```python
from build123d import *

# Parameters (mm, degrees)
SKETCH_1_W          = 20
SKETCH_1_H          = 12
SKETCH_1_R          = 1.25
SKETCH_1_R_2        = 0.6
SKETCH_1_R_3        = 2.6
EXTRUDE_1_DEPTH     = 2.8
EXTRUDE_START       = 2.8
SKETCH_1_9_W        = 20
SKETCH_1_9_H        = 12
SKETCH_1_9_R        = 1.25
EXTRUDE_2_DEPTH     = 0.5
EXTRUDE_START_2     = 3.3
SKETCH_1_10_W       = 20
SKETCH_1_10_H       = 12
SKETCH_1_10_R       = 1.25
SKETCH_1_10_R_2     = 2.6
EXTRUDE_3_DEPTH     = 2.8
SKETCH_3_R          = 0.75
SKETCH_3_R_2        = 0.35
CUT_EXTRUDE_3_DEPTH = 25.108297327
CUT_EXTRUDE_START   = 6.1
SKETCH_3_4_R        = 1
CUT_EXTRUDE_5_DEPTH = 5.1


with BuildPart() as part:
    # 草图1 → 凸台-拉伸1 (new body)
    with BuildSketch(Plane(origin=(0, 0, 0), x_dir=(1, 0, 0), z_dir=(0, 1, 0))):
        with Locations((10, -6)):
            Rectangle(SKETCH_1_W, SKETCH_1_H)
        with Locations(Location((15, -6, 0), (0, 0, 270))):
            Circle(SKETCH_1_R, mode=Mode.SUBTRACT)
        with Locations(Location((7.678736094, -8.970584613, 0), (0, 0, 270))):
            Circle(SKETCH_1_R_2, mode=Mode.SUBTRACT)
        with Locations(Location((9.847079862, -3.807418404, 0), (0, 0, 270))):
            Circle(SKETCH_1_R_3, mode=Mode.SUBTRACT)
    extrude(amount=EXTRUDE_1_DEPTH)

    # 草图1<9> → 凸台-拉伸2 (add)
    with BuildSketch(Plane(origin=(0, 0, 0), x_dir=(1, 0, 0), z_dir=(0, 1, 0)).offset(EXTRUDE_START)):
        with Locations((10, -6)):
            Rectangle(SKETCH_1_9_W, SKETCH_1_9_H)
        with Locations(Location((15, -6, 0), (0, 0, 270))):
            Circle(SKETCH_1_9_R, mode=Mode.SUBTRACT)
    extrude(amount=EXTRUDE_2_DEPTH)

    # 草图1<10> → 凸台-拉伸3 (add)
    with BuildSketch(Plane(origin=(0, 0, 0), x_dir=(1, 0, 0), z_dir=(0, 1, 0)).offset(EXTRUDE_START_2)):
        with Locations((10, -6)):
            Rectangle(SKETCH_1_10_W, SKETCH_1_10_H)
        with Locations(Location((15, -6, 0), (0, 0, 270))):
            Circle(SKETCH_1_10_R, mode=Mode.SUBTRACT)
        with Locations(Location((9, -6, 0), (0, 0, 270))):
            Circle(SKETCH_1_10_R_2, mode=Mode.SUBTRACT)
    extrude(amount=EXTRUDE_3_DEPTH)

    # 草图3 → 切除-拉伸3 (cut, through all)
    with BuildSketch(Plane(origin=(0, 0, 0), x_dir=(1, 0, 0), z_dir=(0, 1, 0))):
        with Locations(Location((1.5, -1.5, 0), (0, 0, 270))):
            Circle(SKETCH_3_R)
        with Locations(Location((1.5, -10.5, 0), (0, 0, 270))):
            Circle(SKETCH_3_R)
        with Locations(Location((18.5, -10.5, 0), (0, 0, 270))):
            Circle(SKETCH_3_R)
        with Locations(Location((18.5, -1.5, 0), (0, 0, 270))):
            Circle(SKETCH_3_R)
        with Locations(Location((2, -6, 0), (0, 0, 270))):
            Circle(SKETCH_3_R_2)
        with Locations(Location((14, -1.5, 0), (0, 0, 270))):
            Circle(SKETCH_3_R_2)
        with Locations(Location((14, -10.5, 0), (0, 0, 270))):
            Circle(SKETCH_3_R_2)
    extrude(amount=CUT_EXTRUDE_3_DEPTH, mode=Mode.SUBTRACT)

    # 草图3<4> → 切除-拉伸5 (cut)
    with BuildSketch(Plane(origin=(0, 0, 0), x_dir=(1, 0, 0), z_dir=(0, 1, 0)).offset(CUT_EXTRUDE_START)):
        with Locations(Location((1.5, -1.5, 0), (0, 0, 270))):
            Circle(SKETCH_3_4_R)
        with Locations(Location((1.5, -10.5, 0), (0, 0, 270))):
            Circle(SKETCH_3_4_R)
        with Locations(Location((18.5, -1.5, 0), (0, 0, 270))):
            Circle(SKETCH_3_4_R)
        with Locations(Location((18.5, -10.5, 0), (0, 0, 270))):
            Circle(SKETCH_3_4_R)
    extrude(amount=-CUT_EXTRUDE_5_DEPTH, mode=Mode.SUBTRACT)


solid = part.part
```
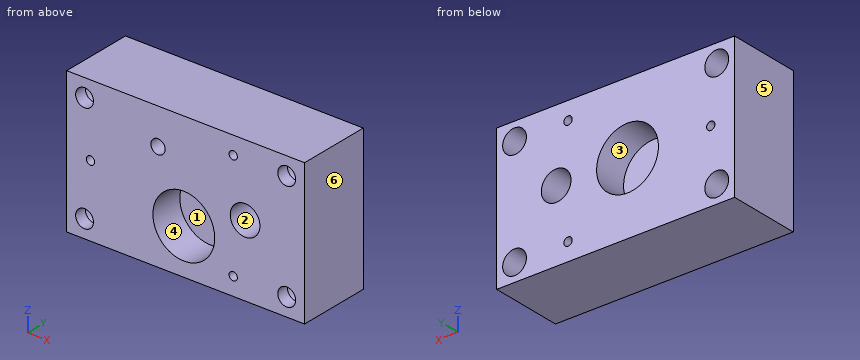
The listing builds one solid part. Answer for the finished solid, in the listing's coordinates (mm). Face numbers are marked on the shaded views. A direction names the side the tool comes from. Give positions to 0.01 mm unless a question says otherwise; leave off trailing zeros. Order: outer loops, then holes, each group sorted by start corner. A loop starts at its lowest first (then second) coordinate and runs counter-clockwise, first axis right, second up. Notation, with made-up numbers: (69, 45.5) - (98, 45.5) arc R15 cw to (98, 66.5) - close; hole circle Ø9 at (10, 27.25). An arc over 180 degrees is marked (long way). Use one line per item in the form item = value. Start each with the question number.
(1) A cutting plane is placed at A-A, the plane z = 1.5. Write down the section's boundary in (x, y), then the cut area to 3 significant figures.
(2) A cutting plane is placed at B-B, the plane x = 15.25. Write down the section's boundary in (y, z), then the cut area to 3 significant figures.
(3) For the marked faces 1, 2 and 3, determine the directions among +Z, -Z, +X, -X, +Y, -Y from which every point of the face is accessible in a straight line to the end or side of a thin tool.
(4) Consider line 1 (Z direction, x = 1.5, y = 0.75); line 2 (X direction, y = 4.65, z = 1.5); line 3 (X direction, y = 0.5, z = 10.5). Determine where each line is inside the solid, lowest interval first. Write a range as from..to.
(5) The mould has two halves that part along X. Classify the marked faces 4, 5 and 6: released by +X, released by -X, zero draft, split by the parting line, or undercut.
(6) Flat-ended cylindrical pins translate along their axes: pin 1 Ø3 at (x, z) = (9, 6) entering from +Y; pin 2 Ø2 at (x, z) = (1.5, 11) entering from +Y; pin 3 Ø1.6 at (x, z) = (18.5, 1.5) entering from +Y. Find the tip coordinate at first contact, or state that the pin passes through.
(7) A cutting plane is placed at C-C, the plane y = 3.75. State how many separate pieces and enclosed holes the cut face has, then the cut area to 3 significant figures.
Ans:
q1.outline = (0, 0) - (0.75, 0) - (0.75, 1) - (0.5, 1) - (0.5, 6.1) - (0, 6.1) - close; (2.25, 0) - (8.65, 0) - (8.65, 2.8) - (11.05, 2.8) - (11.05, 0) - (13.65, 0) - (13.65, 6.1) - (2.5, 6.1) - (2.5, 1) - (2.25, 1) - close; (14.35, 0) - (17.75, 0) - (17.75, 1) - (17.5, 1) - (17.5, 6.1) - (14.35, 6.1) - close; (19.25, 0) - (20, 0) - (20, 6.1) - (19.5, 6.1) - (19.5, 1) - (19.25, 1) - close
q1.area = 87.6 mm^2
q2.outline = (0, 0) - (6.1, 0) - (6.1, 4.78) - (0, 4.78) - close; (0, 7.22) - (6.1, 7.22) - (6.1, 12) - (0, 12) - close
q2.area = 58.3 mm^2
q3.face_1 = -Y
q3.face_2 = +Y, -Y
q3.face_3 = +Y
q4.line_1 = 0..0.75, 2.25..9.75, 11.25..12
q4.line_2 = 0..0.5, 2.5..13.65, 14.35..17.5, 19.5..20
q4.line_3 = 0..0.75, 2.25..13.65, 14.35..17.75, 19.25..20
q5.face_4 = undercut
q5.face_5 = released by -X
q5.face_6 = released by +X
q6.pin_1 = 3.3
q6.pin_2 = 6.1
q6.pin_3 = 1
q7.separate_pieces = 1
q7.enclosed_holes = 9
q7.area = 200 mm^2
